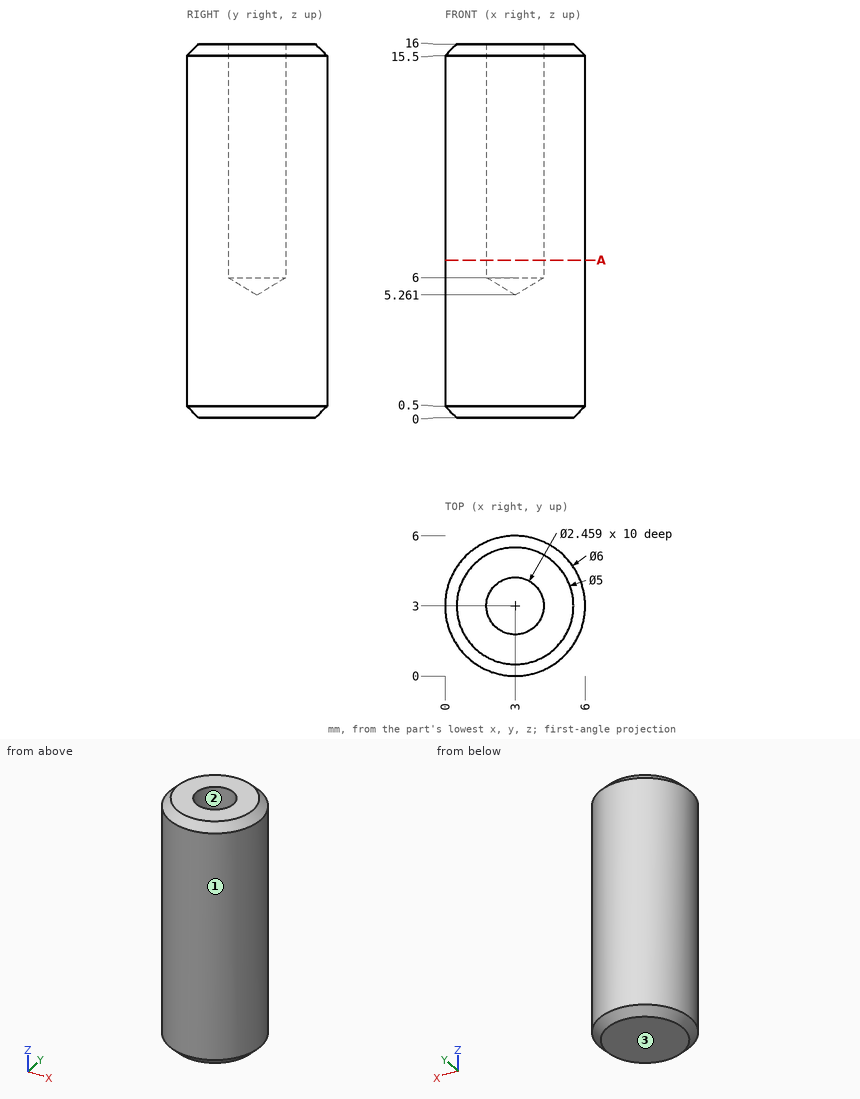
Geometry check sheet. Reference: drawing and pictorial views, mm from the part's lowest x, y, z. Round coordinates to 2 decimals unless told otherwise and drop trailing zeros. Order: outer loops, then holes, each group sorted by start corner. A loop starts at its lowest first (then second) coordinate and runs counter-clockwise, first axis right, second up. Notation, with made-up numbers: (60, 6) - (116, 6) arc R26 ccw to (116, 30) - close; hole circle Ø2 at (79.25, -38). An arc over 180 degrees is marked (long way). Write item = value, one per line.
Q1. Thickness scan on line 1 along Y through (x, z) = (3, 12.25); line 2 along Y through (x, z) = (4, 13.25) (1 decimal); line 3 along Y through (x, z) = (1.7, 9.75). Record the ranges inside material, lowest first.
Computed:
line_1 = 0 to 1.77, 4.23 to 6
line_2 = 0.2 to 2.3, 3.7 to 5.8
line_3 = 0.3 to 5.7
Q2. Draft check along X on the marked faces 1, 2 and 3. Enter one of: pulls with the +X half, pulls with the -X half, needs draft (parallel to the pull), parting line crosses it, or undercut.
Computed:
face_1 = parting line crosses it
face_2 = undercut
face_3 = needs draft
Q3. Section check A-A (z = 6.75). Record the boundary of the cut face in (x, y), and give its area (3 significant figures).
Computed:
outline = circle Ø6 at (3, 3); hole circle Ø2.46 at (3, 3)
area = 23.5 mm^2
Q4. Go/stop test with a flat-tipped pin: pin 1 (2 mm diameter, centred on y = 3.5, z = 13.5, fed in from +X). Record where the tip stops, or that it passes through.
Computed:
pin_1 = 6
